```python
from build123d import *

# Parameters (mm, degrees)
F0_W      = 56
F0_H      = 64
F1_DEPTH  = 8
F2_W      = 8
F2_H      = 50
F3_DEPTH  = 28
F4_R      = 8
F5_DEPTH  = 8
F6_R      = 5
F7_DEPTH  = 8.001
F8_W      = 40
F8_H      = 36
F9_DEPTH  = 17
F10_R     = 11
F11_DEPTH = 25.001


# Not quite as in the source:
# - a pattern or mirror of a feature is missing from the dataset's text; its kind, count and spacing are read off the source's solid


with BuildPart() as f1:
    # F0 (on Top) → F1 (new body)
    with BuildSketch(Plane.XY):
        Rectangle(F0_W, F0_H)
    extrude(amount=-F1_DEPTH)

    # F2 (on face) → F3 (join)
    with BuildSketch(Plane.XY):
        with Locations((-24, 0)):
            Rectangle(F2_W, F2_H)
    f3 = extrude(amount=F3_DEPTH)

    # F3_copies: F3 across plane
    add(f3.mirror(Plane(origin=(0, 0, 0), x_dir=(0, 0, 1), z_dir=(1, 0, 0))))

    # F4 (on face) → F5 (join, through all)
    with BuildSketch(Plane.XY):
        with Locations((0, -32)):
            Circle(F4_R)
    f5 = extrude(amount=-F5_DEPTH)

    # F5_copies: F5 across plane
    add(f5.mirror(Plane.ZX))

    # F6 (on face) → F7 (cut, through all)
    with BuildSketch(Plane.XY):
        with Locations((0, -32)):
            Circle(F6_R)
    f7 = extrude(amount=-F7_DEPTH, mode=Mode.SUBTRACT)

    # F7_copies: F7 across plane
    add(f7.mirror(Plane.ZX), mode=Mode.SUBTRACT)

    # F8 (on face) → F9 (join)
    with BuildSketch(Plane.XY):
        Rectangle(F8_W, F8_H)
    extrude(amount=F9_DEPTH)

    # F10 (on face) → F11 (cut, through all)
    with BuildSketch(Plane.XY.offset(17)):
        Circle(F10_R)
    extrude(amount=-F11_DEPTH, mode=Mode.SUBTRACT)


solid = f1.part
```
Input: part model. Units: mm. Frame: model coordinates. A direction names the side the tool comes from. Give positions to 0.01 mm unless a question says otherwise; leave off trailing zeros. Order: outer loops, then holes, each group sorted by start corner. A loop starts at its lowest first (then second) coordinate and runs counter-clockwise, first axis right, second up.
1. Line query: probe 1 along Y at (x, z) = (0, -5.25); probe 2 along X at (y, z) = (-19, 15); probe 3 along Y at (x, z) = (25.5, 1). Output: solid intervals per line, ascending.
Computed:
probe 1: y = -40 to -37, -27 to -11, 11 to 27, 37 to 40
probe 2: x = -28 to -20, 20 to 28
probe 3: y = -25 to 25
2. Set-up query: faces 4 (the face through (18, -32, -4)), 5 (the face through (24, -25, 14)), 6 (the face through (24, 25, 14)). Return all of +Z, -Z, +X, -X, +Y, -Y with unobstructed straight access to the full face (end or side cutting, diameter ignored); none if empty.
Computed:
face 4: +Z, -Z, +X, -Y
face 5: +Z, +X, -X, -Y
face 6: +Z, +X, -X, +Y
3. Pin query (flat end, axial travel): pin 1 Ø9 at (x, y) = (0, -32) entering from -Z; pin 2 Ø9 at (x, z) = (15.5, -3) entering from +Y; pin 3 Ø6.5 at (x, z) = (24.5, 15.5) entering from -Y; pin 4 Ø18 at (x, y) = (-0.5, 2) entering from +Z. Return the tip coordinate at first contact, or that it passes through.
Computed:
pin 1: passes through
pin 2: stops at y = 32
pin 3: stops at y = -25
pin 4: stops at z = 17
4. Cut plane D-D (z = 25). Return loops of the section in (x, y).
Computed:
outline: (-28, -25) - (-20, -25) - (-20, 25) - (-28, 25) - close; (20, -25) - (28, -25) - (28, 25) - (20, 25) - close
5. Cut plane B-B (z = 6). Return loops of the section in (x, y), and give its area (3 significant figures).
Computed:
outline: (-28, -25) - (-20, -25) - (-20, -18) - (20, -18) - (20, -25) - (28, -25) - (28, 25) - (20, 25) - (20, 18) - (-20, 18) - (-20, 25) - (-28, 25) - close; hole circle Ø22 at (0, 0)
area: 1,860 mm2
6. Draft query along X for faces 1 (the face through (24, 0, 28)), 2 (the face through (0, 18, 8)), 3 (the face through (0, -40, -4)). Return one class per face: released by +X, released by -X, zero draft, split by the parting line, or undercut.
Computed:
face 1: zero draft
face 2: undercut
face 3: split by the parting line
7. Cut plane C-C (x = 0). Return loops of the section in (y, z), and give its area (3 significant figures).
Computed:
outline: (-40, -8) - (-37, -8) - (-37, 0) - (-40, 0) - close; (-27, -8) - (-11, -8) - (-11, 17) - (-18, 17) - (-18, 0) - (-27, 0) - close; (11, -8) - (27, -8) - (27, 0) - (18, 0) - (18, 17) - (11, 17) - close; (37, -8) - (40, -8) - (40, 0) - (37, 0) - close
area: 542 mm2
8. Cut plane A-A (y = 0). Return loops of the section in (x, z), and give its area (3 significant figures).
Computed:
outline: (-28, -8) - (-11, -8) - (-11, 17) - (-20, 17) - (-20, 28) - (-28, 28) - close; (11, -8) - (28, -8) - (28, 28) - (20, 28) - (20, 17) - (11, 17) - close
area: 1,030 mm2
